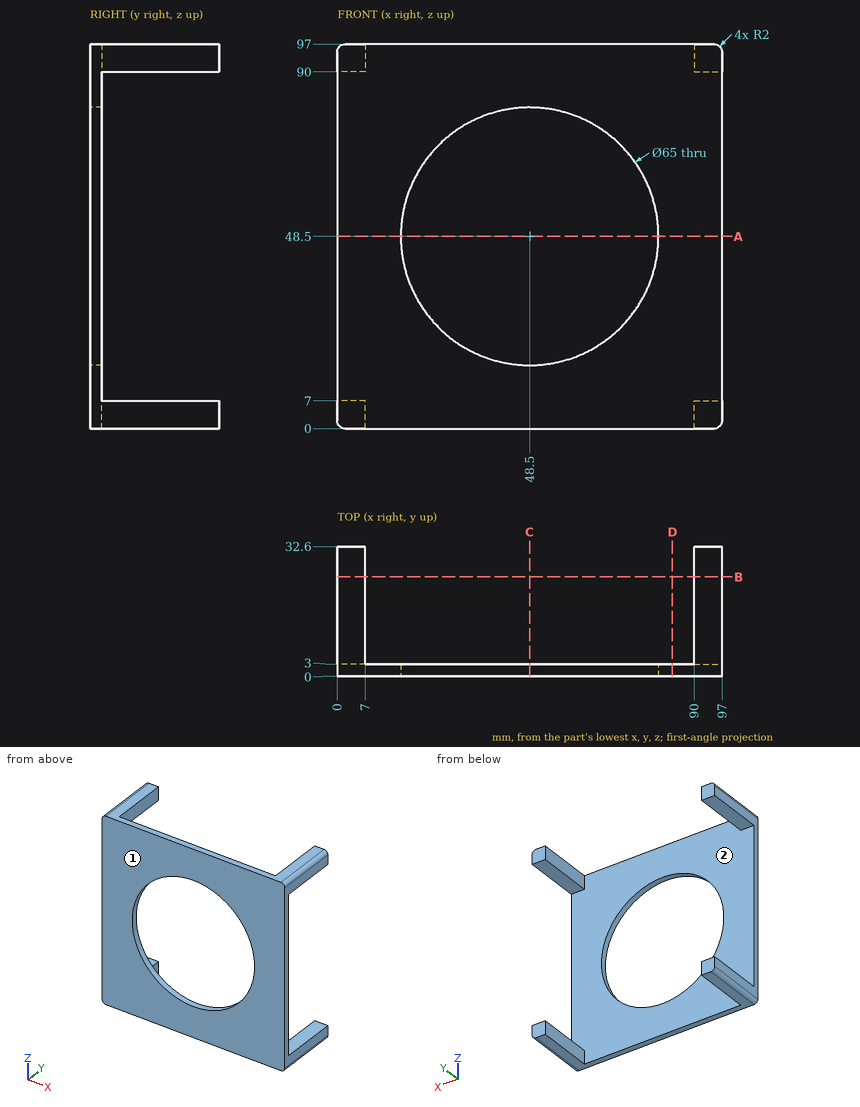
Study the drawing (mm; zero at the part's minimum x, y, z) and answer. Coordinates: 2 decimals unless noted, no trailing zeros. Write each loop counter-clockwise with the first axis right and the second up, starting at its lowest first coordinate (ties: lowest second). Pieces come first, ordered by that corner, then holes. Notation, with made-up numbers: M 87,1.25 L 105,1.25 A20 ccw 105,5.25 Z; hole C 39.25,58 d9. An arc over 180 degrees is marked long. Use a Markdown table: item, result. Add a question column.
1. Section A-A (z = 48.5) is taken. Give the vertices of the cut face in (x, y), plus the area to 3 significant figures.
2. Section D-D (x = 84.5) is taken. Give the vertices of the cut face in (y, z).
3. Section B-B (y = 25) is taken. Give the vertices of the cut face in (x, z).
4. Straight lines are drawn through the part: line 1 along Z through (x, y) = (48.5, 0.85); line 2 along Y through (x, z) = (30, 6). For each, find the intervals that lie inside material, in ascending order. Write a range as [from, to].
5. Section C-C (x = 48.5) is taken. Give the vertices of the cut face in (y, z).
6. For a pull along X with two mould halves and no side action, classify the marked faces 1 and 2 as +X half, -X half, draft (parallel to the pull), parting line (faces both ways), or undercut.
7. Given P1, Ø3.5, axis at x = 3, y = 25, coming from the -Z side; P2, Ø5, axis at x = 42.5, y = 6.5, coming from the -Z side; P3, Ø5, axis at x = 16, z = 24.5, coming from the +Y side, each flat-ended and moving along its own axis, determine where each tip first touches the part or whether it passes through.
Data:
| question | item | result |
|---|---|---|
| 1 | outline | M 0,0 L 16,0 L 16,3 L 0,3 Z; M 81,0 L 97,0 L 97,3 L 81,3 Z |
| 1 | area | 96.0 mm2 |
| 2 | outline | M 0,0 L 3,0 L 3,97 L 0,97 Z |
| 3 | outline | M 0,2 A2 ccw 2,0 L 7,0 L 7,7 L 0,7 Z; M 0,90 L 7,90 L 7,97 L 2,97 A2 ccw 0,95 Z; M 90,0 L 95,0 A2 ccw 97,2 L 97,7 L 90,7 Z; M 90,90 L 97,90 L 97,95 A2 ccw 95,97 L 90,97 Z |
| 4 | line 1 | z = [0, 16], [81, 97] |
| 4 | line 2 | y = [0, 3] |
| 5 | outline | M 0,0 L 3,0 L 3,16 L 0,16 Z; M 0,81 L 3,81 L 3,97 L 0,97 Z |
| 6 | face 1 | draft |
| 6 | face 2 | undercut |
| 7 | P1 | stops at z = 0 |
| 7 | P2 | passes through |
| 7 | P3 | stops at y = 3 |
